The model under review builds one solid part; all positions refer to its coordinate system, in mm. Face numbers are marked on the shaded views. A direction names the side the tool comes from. Coordinates: 2 decimals unless noted, no trailing zeros. Loops run counter-clockwise (first coordinate to the right, second up) from the corner with the lowest first, then second, coordinate; pieces in that order, holes last. Notation, with made-up numbers: (11.25, -5) - (62.25, -5) arc R19 cw to (62.25, 21) - close; hole circle Ø10 at (78, -27). An arc over 180 degrees is marked (long way). Answer in a Markdown table with one row per item. Add a question column.
(1) We need section C-C on x = 4. Write out the cut boundary in (y, z) (3 decimals).
(2) We need section A-A on z = 0. Write out the cut boundary in (x, y).
(3) We need section B-B on y = 18.5. Write out the cut boundary in (x, z), plus the area to 3 significant figures.
(4) For line 1 along Y through (x, z) = (12, 0); line 2 along Y through (x, z) = (43, -21.5); line 3 along Z through (x, y) = (24, 2), list the stretches that pass through material, from the lowest coordinate up.
(5) For P1, Ø8, axis at x = 10.5, z = 28, coming from the +Y side; P2, Ø13.5, axis at x = 34, z = 22.5, coming from the -Y side; P3, Ø12, axis at x = 41, z = -15, coming from the -Y side, all flat-tipped, find the tip position at first contact; note any pin that passes through.
(6) Mouldability with a two-part tool opening along Y and no side actions: class the marked faces 4, 5, 6 and 7 as +Y half, -Y half, draft (parallel to the pull), parting line (faces both ways), or undercut.
(7) We need section D-D on z = 18.5. Write out the cut boundary in (x, y).
(8) Machinability: for the marked faces 1, 2 and 3, which of the approach directions +Z, -Z, +X, -X, +Y, -Y give a long, thin tool a straight path to every point of the face, cutting with its end or side? Answer none if there is none.
from build123d import *

# Parameters (mm, degrees)
BOSS_EXTRUDE1_DEPTH = 47.9


with BuildPart() as part:
    # Sketch1 → Boss-Extrude1 (new body)
    with BuildSketch(Plane(origin=(0, 0, 0), x_dir=(0, 0, -1), z_dir=(1, 0, 0))):
        with BuildLine():
            Line((-15, 0), (-42, 0))
            Line((-42, 0), (-42, 26.5))
            Line((-42, 26.5), (-32.65, 26.5))
            Line((-32.65, 26.5), (-32.65, 25))
            Line((-32.65, 25), (-39.775, 25))
            Line((-39.775, 25), (-39.775, 20))
            Line((-39.775, 20), (-12.75, 20))
            Line((-12.75, 20), (-12.75, 8.865100112))
            ThreePointArc((-12.75, 8.865100112), (0, 15.529085614), (12.75, 8.865100112))
            Line((12.75, 8.865100112), (12.75, 20))
            Line((12.75, 20), (39.775, 20))
            Line((39.775, 20), (39.775, 25))
            Line((39.775, 25), (32.65, 25))
            Line((32.65, 25), (32.65, 26.5))
            Line((32.65, 26.5), (42, 26.5))
            Line((42, 26.5), (42, 0))
            Line((42, 0), (15, 0))
            ThreePointArc((15, 0), (0, -15), (-15, 0))
        make_face()
        with BuildLine():
            ThreePointArc((-12.75, 0), (0, -12.75), (12.75, 0))
            ThreePointArc((12.75, 0), (0, 12.75), (-12.75, 0))
        make_face(mode=Mode.SUBTRACT)
    extrude(amount=BOSS_EXTRUDE1_DEPTH)


solid = part.part
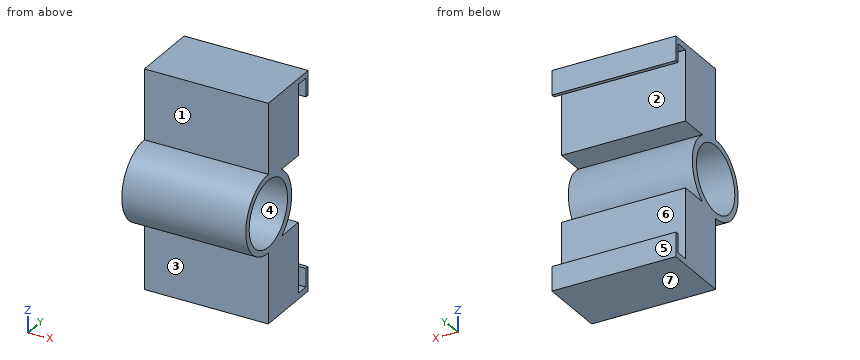
Outcome:
| question | item | result |
|---|---|---|
| 1 | outline | (0, -42) - (26.5, -42) - (26.5, -32.65) - (25, -32.65) - (25, -39.775) - (20, -39.775) - (20, -12.75) - (8.865, -12.75) arc R15.529 ccw to (8.865, 12.75) - (20, 12.75) - (20, 39.775) - (25, 39.775) - (25, 32.65) - (26.5, 32.65) - (26.5, 42) - (0, 42) - (0, 15) arc R15 ccw to (0, -15) - close; hole circle Ø25.5 at (0, 0) |
| 2 | outline | (0, -15) - (47.9, -15) - (47.9, -12.75) - (0, -12.75) - close; (0, 12.75) - (47.9, 12.75) - (47.9, 15.53) - (0, 15.53) - close |
| 3 | outline | (0, -42) - (47.9, -42) - (47.9, -12.75) - (0, -12.75) - close; (0, 12.75) - (47.9, 12.75) - (47.9, 42) - (0, 42) - close |
| 3 | area | 2,800 mm² |
| 4 | line 1 | -15 to -12.75, 12.75 to 15.53 |
| 4 | line 2 | 0 to 20 |
| 4 | line 3 | -42 to -12.59, 12.59 to 42 |
| 5 | P1 | y = 20 |
| 5 | P2 | y = 0 |
| 5 | P3 | y = -12 |
| 6 | face 4 | undercut |
| 6 | face 5 | +Y half |
| 6 | face 6 | undercut |
| 6 | face 7 | draft |
| 7 | outline | (0, 0) - (47.9, 0) - (47.9, 20) - (0, 20) - close |
| 8 | face 1 | +Z, +X, -X, -Y |
| 8 | face 2 | +X, -X |
| 8 | face 3 | -Z, +X, -X, -Y |
